Design review of the part built by this model. Coordinates are the model's own, in mm. Face numbers are marked on the shaded views. A direction names the side the tool comes from. Round coordinates to 2 decimals unless told otherwise and drop trailing zeros. Loops run counter-clockwise (first coordinate to the right, second up) from the corner with the lowest first, then second, coordinate; pieces in that order, holes last. Notation, with made-up numbers: M -6.75,30.5 L 28.25,30.5 A25 cw 28.25,46.5 Z; hole C 87.5,62 d4. An arc over 180 degrees is marked long. Use a Markdown table: item, result.
from build123d import *

# Parameters (mm, degrees)
SKETCH_1_R               = 11
EXTRUDE_1_DEPTH          = 18
EXTRUDE_2_DEPTH          = 18
FILLET_1_R               = 2
CUT_EXTRUDE_1_DEPTH      = 54.23509778
CUT_EXTRUDE_1_DEPTH_BACK = 54.23509778
SKETCH_3_W               = 20
SKETCH_3_H               = 8.1
SKETCH_4_R               = 3
CUT_EXTRUDE_2_DEPTH      = 4.95
SKETCH_5_R               = 2.1
CUT_EXTRUDE_3_DEPTH      = 54.23509778
FILLET_2_R               = 7


with BuildPart() as part:
    # Эскиз1 → Бобышка-Вытянуть1 (new body)
    with BuildSketch(Plane.XY):
        Circle(SKETCH_1_R)
    extrude(amount=EXTRUDE_1_DEPTH)

    # Эскиз2 → Бобышка-Вытянуть2 (add)
    with BuildSketch(Plane.XY):
        with BuildLine():
            Line((48.76838274, 3.610991898), (48.76838274, 2.595691289))
            ThreePointArc((48.76838274, 2.595691289), (47.88840056, 0.473069222), (45.76469978, -0.40430645))
            Line((45.76469978, -0.40430645), (38.399722319, 2.422654444))
            ThreePointArc((38.399722319, 2.422654444), (24.484941772, 5.325401982), (10.366167345, 3.680023719))
            Line((10.366167345, 3.680023719), (-0.971178616, 10.957043949))
            ThreePointArc((-0.971178616, 10.957043949), (23.009820936, 10.8960239), (46.584150264, 6.497949353))
            ThreePointArc((46.584150264, 6.497949353), (48.160798106, 5.421060602), (48.76838274, 3.610991898))
        make_face()
    extrude(amount=EXTRUDE_2_DEPTH)

    # Скругление1
    fillet_1_edges = [part.edges().sort_by_distance(p)[0] for p in [
        (45.76469978, -0.40430645, 9),
    ]]
    fillet(fillet_1_edges, radius=FILLET_1_R)

    # Эскиз3 → Вырез-Вытянуть1 (cut, two sides: drawn at the far end of the back side and taken through both)
    with BuildSketch(Plane(origin=(0, 0, 0), x_dir=(1, 0, 0), z_dir=(0, 1, 0)).offset(-CUT_EXTRUDE_1_DEPTH_BACK)):
        with Locations((-1, -9)):
            Rectangle(SKETCH_3_W, SKETCH_3_H)
    extrude(amount=CUT_EXTRUDE_1_DEPTH + CUT_EXTRUDE_1_DEPTH_BACK, mode=Mode.SUBTRACT)

    # Эскиз4 → Вырез-Вытянуть2 (cut)
    with BuildSketch(Plane.XY.offset(18)):
        with Locations((0, 3)):
            Circle(SKETCH_4_R)
    extrude(amount=-CUT_EXTRUDE_2_DEPTH, mode=Mode.SUBTRACT)

    # Эскиз5 → Вырез-Вытянуть3 (cut, through all)
    with BuildSketch(Plane.XY.offset(18)):
        with Locations((0, 3)):
            Circle(SKETCH_5_R)
    extrude(amount=-CUT_EXTRUDE_3_DEPTH, mode=Mode.SUBTRACT)

    # Скругление2
    fillet_2_edges = [part.edges().sort_by_distance(p)[0] for p in [
        (10.366167345, 3.680023719, 9),
    ]]
    fillet(fillet_2_edges, radius=FILLET_2_R)


solid = part.part
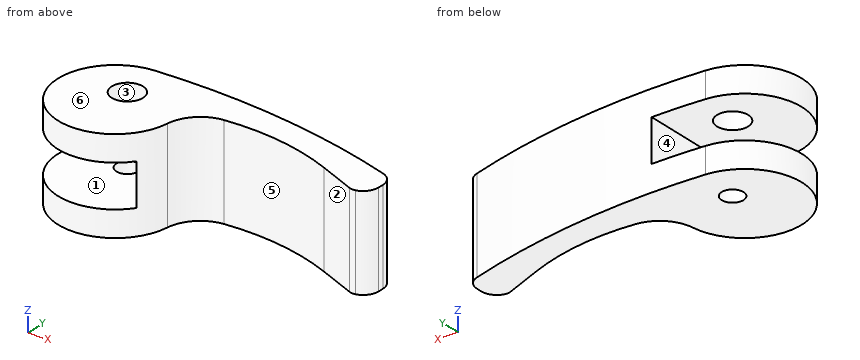
1. Take a section at B-B on y = -4.5. Give the boundary of the cut face in (x, z), and give its area (3 significant figures).
Check values:
| item | result |
|---|---|
| outline | M -10.04,0 L 10.04,0 L 10.04,18 L -10.04,18 L -10.04,13.05 L 9,13.05 L 9,4.95 L -10.04,4.95 Z |
| area | 207 mm² |
2. The part is to be moulded in two halves that separate along Z. For the marked faces 4, 5 and 6, say which applies: pulls with the +Z half, pulls with the -Z half, needs draft (parallel to the pull), parting line crosses it, or undercut.
Check values:
| item | result |
|---|---|
| face 4 | undercut |
| face 5 | needs draft |
| face 6 | pulls with the +Z half |
3. Insertion check: pin 1 (3 mm diameter, centred on y = -5.5, z = 8, fed in from -X); pin 2 (3 mm diameter, centred on x = 6, z = 12, fed in from -Y); pin 3 (1.5 mm diameter, centred on y = 4.5, z = 4, fed in from +X); pin 4 (3 mm diameter, centred on y = -8.5, z = 9.5, fed in from +X). Each pin has a flat end and moves straight along its axis. Give the tip position at first contact, or say it passes through.
Check values:
| item | result |
|---|---|
| pin 1 | stops at x = 9 |
| pin 2 | stops at y = -9.83 |
| pin 3 | stops at x = 48.77 |
| pin 4 | passes through |
4. Take a section at D-D on y = 8.5. Give the boundary of the cut face in (x, z), and give its area (3 significant figures).
Check values:
| item | result |
|---|---|
| outline | M -6.98,0 L 38.54,0 L 38.54,18 L -6.98,18 L -6.98,13.05 L 9,13.05 L 9,4.95 L -6.98,4.95 Z |
| area | 690 mm² |
5. Machinability: for the marked faces 1, 2 and 3, which of the approach directions +Z, -Z, +X, -X, +Y, -Y give a long, thin tool a straight path to every point of the face, cutting with its end or side? Answer none if there is none.
Check values:
| item | result |
|---|---|
| face 1 | -X, +Y, -Y |
| face 2 | +Z, -Z, -Y |
| face 3 | +Z |
6. Take a section at A-A on x = 0. Give the boundary of the cut face in (y, z).
Check values:
| item | result |
|---|---|
| outline | M -11,0 L 0.9,0 L 0.9,4.95 L -11,4.95 Z; M -11,13.05 L 0,13.05 L 0,18 L -11,18 Z; M 5.1,0 L 11.04,0 L 11.04,4.95 L 5.1,4.95 Z; M 6,13.05 L 11.04,13.05 L 11.04,18 L 6,18 Z |
7. Take a section at C-C on x = 7. Give the boundary of the cut face in (y, z).
Check values:
| item | result |
|---|---|
| outline | M -8.49,0 L 11.42,0 L 11.42,4.95 L -8.49,4.95 Z; M -8.49,13.05 L 11.42,13.05 L 11.42,18 L -8.49,18 Z |
8. Wall thickness on line 1 along Z through (x, y) = (-1.5, 9); line 2 along Y through (x, z) = (0, 2.05): over which ranges is each line inside the solid? List them lowest first. Write a range as from..to.
Check values:
| item | result |
|---|---|
| line 1 | z = 0..4.95, 13.05..18 |
| line 2 | y = -11..0.9, 5.1..11.04 |
